from build123d import *

# Parameters (mm, degrees)
ESTRUSIONE_ESTRUSIONE1_DEPTH = 28
ESTRUSIONE_ESTRUSIONE2_DEPTH = 16
SCHIZZO4_W                   = 16
SCHIZZO4_H                   = 50
ESTRUSIONE_ESTRUSIONE3_DEPTH = 6
ESTRUSIONE_ESTRUSIONE4_DEPTH = 22
FORO_PER_VITE_M4_1_D         = 4.5
FORO_PER_VITE_M4_1_DEPTH     = 30
FORO_PER_VITE_M4_1_TIP       = 1.351936393
FORO_PER_VITE_M4_2_D         = 4.5
FORO_PER_VITE_M4_2_DEPTH     = 30
FORO_PER_VITE_M4_2_TIP       = 1.351936393
SCHIZZO10_W                  = 10
SCHIZZO10_H                  = 5
TAGLIO_ESTRUSIONE1_DEPTH     = 6


with BuildPart() as part:
    # Schizzo2 → Estrusione-Estrusione1 (new body)
    with BuildSketch(Plane.XY):
        Polygon((0, 0), (-10, 0), (-10, -25), (-16, -25), (-16, 25), (-10, 25), (-10, 10), (0, 10), (0, 25), (6, 25), (6, -25), (0, -25), align=None)
    extrude(amount=ESTRUSIONE_ESTRUSIONE1_DEPTH)

    # Schizzo3 → Estrusione-Estrusione2 (add)
    with BuildSketch(Plane(origin=(6, 0, 0), x_dir=(0, 0, -1), z_dir=(1, 0, 0))):
        Polygon((-28, 0), (-38, 0), (-38, -25), (-44, -25), (-44, 25), (-38, 25), (-38, 10), (-28, 10), align=None)
    extrude(amount=-ESTRUSIONE_ESTRUSIONE2_DEPTH)

    # Schizzo4 → Estrusione-Estrusione3 (add)
    with BuildSketch(Plane.ZY.offset(10)):
        with Locations((36, 0)):
            Rectangle(SCHIZZO4_W, SCHIZZO4_H)
    extrude(amount=ESTRUSIONE_ESTRUSIONE3_DEPTH)

    # Schizzo5 → Estrusione-Estrusione4 (add)
    with BuildSketch(Plane(origin=(6, 0, 0), x_dir=(0, 0, -1), z_dir=(1, 0, 0))):
        Polygon((-38, -25), (-44, -25), (-44, 25), (-38, 25), (-38, 5), (-28, 5), (-28, 25), (-22, 25), (-22, -25), (-28, -25), (-28, 0), (-38, 0), align=None)
    extrude(amount=ESTRUSIONE_ESTRUSIONE4_DEPTH)

    # Foro per Vite M4-1
    with Locations(Plane.XY.offset(44)):
        with Locations((18, -20)):
            Hole(FORO_PER_VITE_M4_1_D / 2, depth=FORO_PER_VITE_M4_1_DEPTH)
            with Locations((0, 0, -(FORO_PER_VITE_M4_1_DEPTH + FORO_PER_VITE_M4_1_TIP / 2))):  # 118° drill point
                Cone(0, FORO_PER_VITE_M4_1_D / 2, FORO_PER_VITE_M4_1_TIP, mode=Mode.SUBTRACT)

    # Foro per Vite M4-2
    with Locations(Plane.ZY.offset(16)):
        with Locations((10, -20)):
            Hole(FORO_PER_VITE_M4_2_D / 2, depth=FORO_PER_VITE_M4_2_DEPTH)
            with Locations((0, 0, -(FORO_PER_VITE_M4_2_DEPTH + FORO_PER_VITE_M4_2_TIP / 2))):  # 118° drill point
                Cone(0, FORO_PER_VITE_M4_2_D / 2, FORO_PER_VITE_M4_2_TIP, mode=Mode.SUBTRACT)

    # Schizzo10 → Taglio-Estrusione1 (cut)
    with BuildSketch(Plane(origin=(6, 0, 0), x_dir=(0, 0, -1), z_dir=(1, 0, 0))):
        with Locations((-33, 7.5)):
            Rectangle(SCHIZZO10_W, SCHIZZO10_H)
    extrude(amount=-TAGLIO_ESTRUSIONE1_DEPTH, mode=Mode.SUBTRACT)


solid = part.part
Source: CAD feature listing. Evaluate the final solid. Frame: model axes, mm. A direction names the side the tool comes from. Give positions to 0.01 mm unless a question says otherwise; leave off trailing zeros. Loops run counter-clockwise (first coordinate to the right, second up) from the corner with the lowest first, then second, coordinate; pieces in that order, holes last. Notation, with made-up numbers: (20, 12) -> (65, 12) arc R26 ccw to (65, 37) -> close; hole circle Ø8 at (25.25, 2). An arc over 180 degrees is marked (long way). Use a Markdown table: item, result. Add a question column.
1) Section query B-B, the plane y = -20. Return the cut outline in (x, z), then the cut area to 3 significant figures.
2) Reachability of faces 1 (the face through (17, 0, 22)), 2 (the face through (9, -12, 38)), 3 (the face through (-10, 18, 19)), 4 (the face through (0, -13, 14)), 5 (the face through (14, 5, 33)) from +Z, -Z, +X, -X, +Y, -Y: full face, straight path, thin tool, end or side. Return the list, or none.
3) Section query D-D, the plane y = -10. Return the cut outline in (x, z).
4) First-contact query: pin 1 (1.5 mm diameter, centred on x = -9, z = 33.5, fed in from -Y); pin 2 (5 mm diameter, centred on x = 11.5, y = 12, fed in from -Z); pin 3 (17.5 mm diameter, centred on y = -9.5, z = 12, fed in from +X). Flat tips, straight axial feed; report the tip coordinate or a pass-through.
5) Pull-direction query (Z, two-part tool) for faces 6 (the face through (-5, 10, 19)), 7 (the face through (14, 15, 28)), 8 (the face through (14, -13, 28)), 9 (the face through (-4.8, 0.4, 0)); classes: +Z half, -Z half, draft (parallel to the pull), parting line (faces both ways), or undercut.
6) Line query: line 1 along Z through (x, y) = (25.5, 12); line 2 along X through (y, z) = (-12, 26); line 3 along Y through (x, z) = (18, 39). Output: solid intervals per line, ascending. Write a range as [from, to].
7) Section query C-C, the plane x = 18. Return the cut outline in (y, z), then the cut area to 3 significant figures.
8) Section query A-A, the plane z = 10. Return the cut outline in (x, y).
Numbers:
| question | item | result |
|---|---|---|
| 1 | outline | (-16, 0) -> (-10, 0) -> (-10, 7.75) -> (-16, 7.75) -> close; (-16, 12.25) -> (-10, 12.25) -> (-10, 38) -> (15.75, 38) -> (15.75, 44) -> (-16, 44) -> close; (0, 0) -> (6, 0) -> (6, 7.75) -> (0, 7.75) -> close; (0, 12.25) -> (6, 12.25) -> (6, 22) -> (15.75, 22) -> (15.75, 28) -> (0, 28) -> close; (20.25, 22) -> (28, 22) -> (28, 28) -> (20.25, 28) -> close; (20.25, 38) -> (28, 38) -> (28, 44) -> (20.25, 44) -> close |
| 1 | area | 684 mm2 |
| 2 | face 1 | -Z, +X, +Y, -Y |
| 2 | face 2 | +X, -Y |
| 2 | face 3 | -Z, +Y |
| 2 | face 4 | -Z, -Y |
| 2 | face 5 | +X, +Y |
| 3 | outline | (-16, 0) -> (-10, 0) -> (-10, 38) -> (28, 38) -> (28, 44) -> (-16, 44) -> close; (0, 0) -> (6, 0) -> (6, 22) -> (28, 22) -> (28, 28) -> (0, 28) -> close |
| 4 | pin 1 | stops at y = 0 |
| 4 | pin 2 | stops at z = 22 |
| 4 | pin 3 | stops at x = 6 |
| 5 | face 6 | draft |
| 5 | face 7 | undercut |
| 5 | face 8 | undercut |
| 5 | face 9 | -Z half |
| 6 | line 1 | z = [22, 28], [38, 44] |
| 6 | line 2 | x = [-16, -10], [0, 28] |
| 6 | line 3 | y = [-25, -22.25], [-17.75, 25] |
| 7 | outline | (-25, 22) -> (-22.25, 22) -> (-22.25, 28) -> (-25, 28) -> close; (-25, 38) -> (-22.25, 38) -> (-22.25, 44) -> (-25, 44) -> close; (-17.75, 22) -> (25, 22) -> (25, 28) -> (5, 28) -> (5, 38) -> (25, 38) -> (25, 44) -> (-17.75, 44) -> (-17.75, 38) -> (0, 38) -> (0, 28) -> (-17.75, 28) -> close |
| 7 | area | 596 mm2 |
| 8 | outline | (-16, -25) -> (-10, -25) -> (-10, -22.25) -> (-16, -22.25) -> close; (-16, -17.75) -> (-10, -17.75) -> (-10, 0) -> (0, 0) -> (0, -17.75) -> (6, -17.75) -> (6, 25) -> (0, 25) -> (0, 10) -> (-10, 10) -> (-10, 25) -> (-16, 25) -> close; (0, -25) -> (6, -25) -> (6, -22.25) -> (0, -22.25) -> close |
